from build123d import *

# Parameters (mm, degrees)
F0_W     = 97.335488
F0_H     = 78.626908
F1_DEPTH = 26.924
F2_R     = 15.53957
F3_DEPTH = 25.4
F5_DEPTH = 63.5


with BuildPart() as f1:
    # F0 (on Top) → F1 (new body)
    with BuildSketch(Plane.XY):
        Rectangle(F0_W, F0_H)
    extrude(amount=-F1_DEPTH)

    # F2 (on Top) → F3 (join)
    with BuildSketch(Plane.XY):
        Circle(F2_R)
    extrude(amount=F3_DEPTH)

    # F4 (on Front) → F5 (cut, symmetric)
    with BuildSketch(Plane.XZ):
        Polygon((23.7744, 28.803602), (-18.8976, 28.4988), (23.7744, 0), align=None)
    extrude(amount=F5_DEPTH, both=True, mode=Mode.SUBTRACT)


solid = f1.part
Geometry check sheet. Reference: the model listing, model coordinates, mm. A direction names the side the tool comes from. Coordinates: 2 decimals unless noted, no trailing zeros. Order: outer loops, then holes, each group sorted by start corner. A loop starts at its lowest first (then second) coordinate and runs counter-clockwise, first axis right, second up. Notation, with made-up numbers: (45, -39.75) - (91, -39.75) arc R22 cw to (91, -15.75) - close; hole circle Ø2 at (-15, 36.25). An arc over 180 degrees is marked (long way). Answer in a Markdown table with one row per item. Add a question column.
1) Cross-section at D-D, the plane x = -18.5. Record the cut outline in (y, z).
2) Material ranges on line 1 along Z through (x, y) = (-13, 30.5); line 2 along Y through (x, z) = (-3.5, 4.5); line 3 along Y through (x, z) = (-7.5, 5), recorded low to high. Write a range as [from, to].
3) Gauge pin test, flat ends, axial feed: P1, Ø12, axis at y = -3, z = 19.5, coming from the -X side; P2, Ø5, axis at x = -18, y = -8, coming from the +Z side. Record the tip position at first contact, or that the pin passes through.
4) Cross-section at C-C, the plane z = 9.5. Record the cut outline in (x, y), then the cut area to 3 significant figures.
5) Set-up check for faces 1 (the cylindrical face through (-15.525, 0.683, 9.7)), 2 (the flat face through (-1, -39.313, -13)): record each of +Z, -Z, +X, -X, +Y, -Y from which the full face is reachable in a straight line by a thin tool's end or side.
6) Cross-section at B-B, the plane x = 0. Record the cut outline in (y, z).
7) Cross-section at A-A, the plane y = 0. Record the cut outline in (x, z), then the cut area to 3 significant figures.
Check result:
| question | item | result |
|---|---|---|
| 1 | outline | (-39.31, -26.92) - (39.31, -26.92) - (39.31, 0) - (-39.31, 0) - close |
| 2 | line 1 | z = [-26.92, 0] |
| 2 | line 2 | y = [-15.14, 15.14] |
| 2 | line 3 | y = [-13.61, 13.61] |
| 3 | P1 | stops at x = -15.54 |
| 3 | P2 | stops at z = 0 |
| 4 | outline | (9.55, -12.26) - (9.55, 12.26) arc R15.54 ccw (long way) to start |
| 4 | area | 656 mm² |
| 5 | face 1 | +Z |
| 5 | face 2 | +Z, -Z, +X, -X, -Y |
| 6 | outline | (-39.31, -26.92) - (39.31, -26.92) - (39.31, 0) - (15.54, 0) - (15.54, 15.88) - (-15.54, 15.88) - (-15.54, 0) - (-39.31, 0) - close |
| 7 | outline | (-48.67, -26.92) - (48.67, -26.92) - (48.67, 0) - (15.54, 0) - (15.54, 5.5) - (-14.26, 25.4) - (-15.54, 25.4) - (-15.54, 0) - (-48.67, 0) - close |
| 7 | area | 3,110 mm² |
